```python
from build123d import *

# Parameters (mm, degrees)
EXTRUDE_1_DEPTH          = 78
EXTRUDE_START            = -4
EXTRUDE_1_2_OUTLINE_R    = 2.1
EXTRUDE_1_2_DEPTH        = 4
EXTRUDE_START_2          = -1
EXTRUDE_1_3_OUTLINE_R    = 5
EXTRUDE_1_3_OUTLINE_R_2  = 2.5
EXTRUDE_1_3_DEPTH        = 30
EXTRUDE_START_3          = -25
EXTRUDE_1_4_DEPTH        = 2
EXTRUDE_2_DEPTH          = 2
CUT_EXTRUDE_1_DEPTH      = 98.082439195
FILLET_1_R               = 2
EXTRUDE_START_4          = -2
SKETCH_4_R               = 2.1
SKETCH_4_R_2             = 1
EXTRUDE_3_DEPTH          = 2
HOLE_WIZARD_M4_1_D       = 3.3
HOLE_WIZARD_M4_1_DEPTH   = 11.5
HOLE_WIZARD_M4_1_TIP     = 0.991420021
SKETCH_8_W               = 20
SKETCH_8_H               = 25
CUT_EXTRUDE_2_DEPTH      = 91.498618774
FILLET_2_R               = 2
SKETCH_9_R               = 2.5
SKETCH_9_R_2             = 2.15
EXTRUDE_4_DEPTH          = 2
PATTERN_CIRCULAR_2_COUNT = 3


with BuildPart() as part:
    # ﾎﾞｽ - 押し出し1: read off the stored shape, not the designer's step
    # ﾎﾞｽ - 押し出し1 outline → ﾎﾞｽ - 押し出し1 (new body)
    with BuildSketch(Plane.YZ):
        with BuildLine():
            Line((29, 25), (4, 25))
            ThreePointArc((4, 25), (1.171572875, 23.828427125), (0, 21))
            Line((0, 21), (0, -21))
            ThreePointArc((0, -21), (1.171572875, -23.828427125), (4, -25))
            Line((4, -25), (29, -25))
            Line((29, -25), (29, -23))
            Line((29, -23), (4, -23))
            ThreePointArc((4, -23), (2.585786438, -22.414213562), (2, -21))
            Line((2, -21), (2, 21))
            ThreePointArc((2, 21), (2.585786438, 22.414213562), (4, 23))
            Line((4, 23), (29, 23))
            Line((29, 23), (29, 25))
        make_face()
    extrude(amount=EXTRUDE_1_DEPTH)

    # Extrude 1 2 outline → Extrude 1 2 (add)
    # profile 1 of 2: a face of its own
    with BuildSketch(Plane.YZ.offset(EXTRUDE_START)):
        with BuildLine():
            ThreePointArc((4, 8), (4.228361402, 6.851949703), (4.878679656, 5.878679656))
            ThreePointArc((4.878679656, 5.878679656), (5.851949703, 5.228361402), (7, 5))
            Line((7, 5), (26, 5))
            ThreePointArc((26, 5), (27.148050297, 5.228361402), (28.121320344, 5.878679656))
            ThreePointArc((28.121320344, 5.878679656), (28.771638598, 6.851949703), (29, 8))
            Line((29, 8), (29, 25))
            Line((29, 25), (4, 25))
            Line((4, 25), (4, 8))
        make_face()
        with Locations((9, 15)):
            Circle(EXTRUDE_1_2_OUTLINE_R, mode=Mode.SUBTRACT)
        with Locations((24, 15)):
            Circle(EXTRUDE_1_2_OUTLINE_R, mode=Mode.SUBTRACT)
    # profile 2 of 2: a face of its own
    with BuildSketch(Plane.YZ.offset(EXTRUDE_START)):
        with BuildLine():
            Line((4, -25), (29, -25))
            Line((29, -25), (29, -8))
            ThreePointArc((29, -8), (28.771638598, -6.851949703), (28.121320344, -5.878679656))
            ThreePointArc((28.121320344, -5.878679656), (27.148050297, -5.228361402), (26, -5))
            Line((26, -5), (7, -5))
            ThreePointArc((7, -5), (5.851949703, -5.228361402), (4.878679656, -5.878679656))
            ThreePointArc((4.878679656, -5.878679656), (4.228361402, -6.851949703), (4, -8))
            Line((4, -8), (4, -25))
        make_face()
        with Locations((9, -15)):
            Circle(EXTRUDE_1_2_OUTLINE_R, mode=Mode.SUBTRACT)
        with Locations((24, -15)):
            Circle(EXTRUDE_1_2_OUTLINE_R, mode=Mode.SUBTRACT)
    extrude(amount=EXTRUDE_1_2_DEPTH)

    # Extrude 1 3 outline → Extrude 1 3 (cut)
    with BuildSketch(Plane(origin=(0, 0, 0), x_dir=(1, 0, 0), z_dir=(0, 1, 0)).offset(EXTRUDE_START_2)):
        with Locations((50, 0)):
            Circle(EXTRUDE_1_3_OUTLINE_R)
        with BuildLine():
            Line((0, -5), (-2, -5))
            Line((-2, -5), (-2, -21))
            ThreePointArc((-2, -21), (-1.414213562, -22.414213562), (0, -23))
            Line((0, -23), (0, -5))
        make_face()
        with BuildLine():
            ThreePointArc((0, -25), (-2.828427125, -23.828427125), (-4, -21))
            Line((-4, -21), (-4, -25))
            Line((-4, -25), (0, -25))
        make_face()
        with BuildLine():
            Line((0, 5), (0, 23))
            ThreePointArc((0, 23), (-1.414213562, 22.414213562), (-2, 21))
            Line((-2, 21), (-2, 5))
            Line((-2, 5), (0, 5))
        make_face()
        with BuildLine():
            ThreePointArc((-4, 21), (-2.828427125, 23.828427125), (0, 25))
            Line((0, 25), (-4, 25))
            Line((-4, 25), (-4, 21))
        make_face()
        with Locations((36.004809472, 9.240381057)):
            Circle(EXTRUDE_1_3_OUTLINE_R_2)
        with Locations((48.995190528, -16.740381057)):
            Circle(EXTRUDE_1_3_OUTLINE_R_2)
        with Locations((65, -7.5)):
            Circle(EXTRUDE_1_3_OUTLINE_R_2)
        with Locations((65, 7.5)):
            Circle(EXTRUDE_1_3_OUTLINE_R_2)
        with Locations((36.004809472, -9.240381057)):
            Circle(EXTRUDE_1_3_OUTLINE_R_2)
        with Locations((48.995190528, 16.740381057)):
            Circle(EXTRUDE_1_3_OUTLINE_R_2)
    extrude(amount=EXTRUDE_1_3_DEPTH, mode=Mode.SUBTRACT)

    # Extrude 1 4 outline → Extrude 1 4 (cut)
    with BuildSketch(Plane.XY.offset(EXTRUDE_START_3)):
        with BuildLine():
            ThreePointArc((76.562947136, 7.421535507), (77.140312684, 7.145469965), (77.600920715, 6.701168941))
            ThreePointArc((77.600920715, 6.701168941), (77.89760921, 6.134124767), (78, 5.502397544))
            Line((78, 5.502397544), (78, 29))
            Line((78, 29), (2.712718898, 29))
            ThreePointArc((2.712718898, 29), (2.855262652, 28.994913852), (2.997081408, 28.979681278))
            ThreePointArc((2.997081408, 28.979681278), (3.137453853, 28.954379753), (3.275666034, 28.919137963))
            Line((3.275666034, 28.919137963), (76.562947136, 7.421535507))
        make_face()
    extrude(amount=EXTRUDE_1_4_DEPTH, mode=Mode.SUBTRACT)

    # ｽｹｯﾁ2 → ﾎﾞｽ - 押し出し2 (add)
    with BuildSketch(Plane(origin=(0, 0, -25), x_dir=(-1, 0, 0), z_dir=(0, 0, -1))):
        with BuildLine():
            ThreePointArc((-2.997081408, 28.979681278), (-2.855262652, 28.994913852), (-2.712718898, 29))
            Line((-2.712718898, 29), (-78, 29))
            Line((-78, 29), (-78, 5.502397544))
            ThreePointArc((-78, 5.502397544), (-77.89760921, 6.134124767), (-77.600920715, 6.701168941))
            ThreePointArc((-77.600920715, 6.701168941), (-77.140312684, 7.145469965), (-76.562947136, 7.421535507))
            Line((-76.562947136, 7.421535507), (-3.275666034, 28.919137963))
            ThreePointArc((-3.275666034, 28.919137963), (-3.137453853, 28.954379753), (-2.997081408, 28.979681278))
        make_face()
    extrude(amount=-EXTRUDE_2_DEPTH)

    # ｽｹｯﾁ3 → ｶｯﾄ - 押し出し1 (cut, through all)
    with BuildSketch(Plane.XY.offset(25)):
        Polygon((78, 29), (15, 29), (78, 12), align=None)
    extrude(amount=-CUT_EXTRUDE_1_DEPTH, mode=Mode.SUBTRACT)

    # ﾌｨﾚｯﾄ1
    fillet_1_edges = [part.edges().sort_by_distance(p)[0] for p in [
        (15, 29, -24),
        (78, 12, -24),
        (15, 29, 24),
        (78, 12, 24),
    ]]
    fillet(fillet_1_edges, radius=FILLET_1_R)

    # ｽｹｯﾁ4 → ﾎﾞｽ - 押し出し3 (add)
    # profile 1 of 2: a face of its own
    with BuildSketch(Plane(origin=(-2, 0, 0), x_dir=(0, 0, -1), z_dir=(1, 0, 0)).offset(EXTRUDE_START_4)):
        with Locations((-15, 9)):
            Circle(SKETCH_4_R)
        with Locations(Location((-15, 9, 0), (0, 0, 90))):
            Circle(SKETCH_4_R_2, mode=Mode.SUBTRACT)
    # profile 2 of 2: a face of its own
    with BuildSketch(Plane(origin=(-2, 0, 0), x_dir=(0, 0, -1), z_dir=(1, 0, 0)).offset(EXTRUDE_START_4)):
        with Locations((-15, 24)):
            Circle(SKETCH_4_R)
        with Locations(Location((-15, 24, 0), (0, 0, 90))):
            Circle(SKETCH_4_R_2, mode=Mode.SUBTRACT)
    extrude_3 = extrude(amount=EXTRUDE_3_DEPTH)

    # ﾐﾗｰ2: ﾎﾞｽ - 押し出し3 across plane
    add(extrude_3.mirror(Plane.XY))

    # M4 ねじ穴1
    with Locations(Plane.ZY.offset(4)):
        with Locations((-15, 9), (-15, 24), (15, 24), (15, 9)):
            Hole(HOLE_WIZARD_M4_1_D / 2, depth=HOLE_WIZARD_M4_1_DEPTH)
            with Locations((0, 0, -(HOLE_WIZARD_M4_1_DEPTH + HOLE_WIZARD_M4_1_TIP / 2))):  # 118° drill point
                Cone(0, HOLE_WIZARD_M4_1_D / 2, HOLE_WIZARD_M4_1_TIP, mode=Mode.SUBTRACT)

    # ｽｹｯﾁ8 → ｶｯﾄ - 押し出し2 (cut, through all)
    with BuildSketch(Plane.ZY.offset(4)):
        with Locations((0, 16.5)):
            Rectangle(SKETCH_8_W, SKETCH_8_H)
    extrude(amount=-CUT_EXTRUDE_2_DEPTH, mode=Mode.SUBTRACT)

    # ﾌｨﾚｯﾄ2
    fillet_2_edges = [part.edges().sort_by_distance(p)[0] for p in [
        (-3, 29, 10),
        (-3, 4, 10),
        (-3, 4, -10),
        (-3, 29, -10),
    ]]
    fillet(fillet_2_edges, radius=FILLET_2_R)

    # ｽｹｯﾁ9 → ﾎﾞｽ - 押し出し4 (add)
    # profile 1 of 2: a face of its own
    with BuildSketch(Plane(origin=(0, 2, 0), x_dir=(1, 0, 0), z_dir=(0, 1, 0)).offset(EXTRUDE_START_4)):
        with Locations((48.995190528, 16.740381057)):
            Circle(SKETCH_9_R)
        with Locations(Location((48.995190528, 16.740381057, 0), (0, 0, 270))):
            Circle(SKETCH_9_R_2, mode=Mode.SUBTRACT)
    # profile 2 of 2: a face of its own
    with BuildSketch(Plane(origin=(0, 2, 0), x_dir=(1, 0, 0), z_dir=(0, 1, 0)).offset(EXTRUDE_START_4)):
        with Locations((36.004809472, 9.240381057)):
            Circle(SKETCH_9_R)
        with Locations(Location((36.004809472, 9.240381057, 0), (0, 0, 270))):
            Circle(SKETCH_9_R_2, mode=Mode.SUBTRACT)
    extrude_4 = extrude(amount=EXTRUDE_4_DEPTH)

    # 円形ﾊﾟﾀｰﾝ2: ﾎﾞｽ - 押し出し4 ×3 about axis
    pattern_circular_2_axis = Axis((50, 0, 0), (0, 1, 0))
    for i in range(1, PATTERN_CIRCULAR_2_COUNT):
        add(extrude_4.rotate(pattern_circular_2_axis, i * 360 / PATTERN_CIRCULAR_2_COUNT))


solid = part.part
```
The listing builds one solid part. Answer for the finished solid, in the listing's coordinates (mm). A direction names the side the tool comes from. Round coordinates to 2 decimals unless told otherwise and drop trailing zeros. Loops run counter-clockwise (first coordinate to the right, second up) from the corner with the lowest first, then second, coordinate; pieces in that order, holes last.
Q1. Which of the six approach directions +Z, -Z, +X, -X, +Y, -Y give full straight-line access (tool end or side, diameter ignored) to faces 1 (the face through (-4, 17, 16)), 2 (the face through (40, 2, 0)), 3 (the face through (-3, 16, 10)), 4 (the face through (-2.99, 4.57, -10.6))?
Q2. Section D-D, the plane x = 50 is taken. Determine the outline of the cut face in (y, z), then the cut area to 3 significant figures.
Q3. Given pin 1 Ø4 at (x, z) = (32.5, 5.5) entering from +Y; pin 2 Ø3 at (x, z) = (-3, -17) entering from -Y; pin 3 Ø3.5 at (y, z) = (14, -13) entering from +X, each flat-ended and moving along its own axis, determine where each tip first touches the part or whether it passes through.
Q4. Section B-B, the plane x = 65 is taken. Determine the outline of the cut face in (y, z), then the cut area to 3 significant figures.
Q5. Section A-A, the plane y = 9 is taken. Determine the outline of the cut face in (x, z).
Q6. Section C-C, the plane y = 21 is taken. Determine the outline of the cut face in (x, z).
Q7. For a pull along Y with two mould halves and no side action, classify faces 5 (the face through (-2.986, 8.368, -16.524)), 6 (the face through (-2.986, 8.368, 13.476)), 7 (the face through (-1.43, 16.32, 22.4)), 8 (the face through (-2.99, 28.4, 10.57)) as released by +Y, released by -Y, zero draft, split by the parting line, or undercut.
Q8. Find the intervals of material crossed by line 1 (Y direction, x = -3, z = 15); line 2 (Z direction, x = 13.5, y = 21.75); line 3 (Y direction, x = 71, z = 10), in increasing order.
Completed:
1. face 1: +Z, -Z, -X, +Y, -Y
1. face 2: +X, -X, +Y
1. face 3: +X, -X, +Y, -Y
1. face 4: +X, -X, -Y
2. outline: (0, -21) arc R4 ccw to (4, -25) - (19.56, -25) - (19.56, -23) - (4, -23) arc R2 cw to (2, -21) - (2, -18.64) - (0, -18.64) - close; (0, -14.84) - (2, -14.84) - (2, -5) - (0, -5) - close; (0, 5) - (2, 5) - (2, 14.84) - (0, 14.84) - close; (0, 18.64) - (2, 18.64) - (2, 21) arc R2 cw to (4, 23) - (19.56, 23) - (19.56, 25) - (4, 25) arc R4 ccw to (0, 21) - close
2. area: 130 mm2
3. pin 1: stops at y = 2
3. pin 2: stops at y = 4
3. pin 3: stops at x = -2
4. outline: (0, -21) arc R4 ccw to (4, -25) - (15.51, -25) - (15.51, -23) - (4, -23) arc R2 cw to (2, -21) - (2, -9.65) - (0, -9.65) - close; (0, -5.35) - (2, -5.35) - (2, 5.35) - (0, 5.35) - close; (0, 9.65) - (2, 9.65) - (2, 21) arc R2 cw to (4, 23) - (15.51, 23) - (15.51, 25) - (4, 25) arc R4 ccw to (0, 21) - close
4. area: 132 mm2
5. outline: (-4, -21) arc R4 ccw to (0, -25) - (78, -25) - (78, -23) - (0, -23) arc R2 cw to (-2, -21) - (-2, -16.65) - (-4, -16.65) - close; (-4, -13.35) - (-2, -13.35) - (-2, -10) - (-4, -10) - close; (-4, 10) - (-2, 10) - (-2, 13.35) - (-4, 13.35) - close; (-4, 16.65) - (-2, 16.65) - (-2, 21) arc R2 cw to (0, 23) - (78, 23) - (78, 25) - (0, 25) arc R4 ccw to (-4, 21) - close
6. outline: (-4, -21) arc R4 ccw to (0, -25) - (44.65, -25) - (44.65, -23) - (0, -23) arc R2 cw to (-2, -21) - (-2, -10) - (-4, -10) - close; (-4, 10) - (-2, 10) - (-2, 21) arc R2 cw to (0, 23) - (44.65, 23) - (44.65, 25) - (0, 25) arc R4 ccw to (-4, 21) - close
7. face 5: undercut
7. face 6: undercut
7. face 7: zero draft
7. face 8: released by +Y
8. line 1: y = 4 to 7.35, 10.65 to 22.35, 25.65 to 29
8. line 2: z = -25 to -23, 23 to 25
8. line 3: y = 0 to 2
